from build123d import *

# Parameters (mm, degrees)
EXTRUDE_1_DEPTH     = 5
SKETCH_3_R          = 1.5
CUT_EXTRUDE_1_DEPTH = 5
SKETCH_4_R          = 1.5
CUT_EXTRUDE_2_DEPTH = 50
EXTRUDE_2_DEPTH     = 45
CUT_EXTRUDE_START   = -45
SKETCH_8_R          = 1.5
CUT_EXTRUDE_3_DEPTH = 45


with BuildPart() as part:
    # 草图1 → 凸台-拉伸1 (new body)
    with BuildSketch(Plane(origin=(0, 0, 0), x_dir=(1, 0, 0), z_dir=(0, 1, 0))):
        with BuildLine():
            Line((72.807044649, 44.366167138), (49.314729129, 35.815663555))
            Line((49.314729129, 35.815663555), (49.314729129, 10.486670722))
            Line((49.314729129, 10.486670722), (72.807044649, 1.936167138))
            Line((72.807044649, 1.936167138), (217.807044649, 1.936167138))
            ThreePointArc((217.807044649, 1.936167138), (239.022044649, 23.151167138), (217.807044649, 44.366167138))
            Line((217.807044649, 44.366167138), (72.807044649, 44.366167138))
        make_face()
    extrude(amount=EXTRUDE_1_DEPTH)

    # 草图3 → 切除-拉伸1 (cut)
    with BuildSketch(Plane.XZ):
        with Locations(Location((226.822656109, -14.135555678, 0), (0, 0, 270))):
            Circle(SKETCH_3_R)
        with Locations(Location((224.701335766, -30.045458255, 0), (0, 0, 270))):
            Circle(SKETCH_3_R)
        with Locations(Location((208.791433189, -32.166778599, 0), (0, 0, 270))):
            Circle(SKETCH_3_R)
        with Locations(Location((210.912753532, -16.256876022, 0), (0, 0, 270))):
            Circle(SKETCH_3_R)
    extrude(amount=-CUT_EXTRUDE_1_DEPTH, mode=Mode.SUBTRACT)

    # 草图4 → 切除-拉伸2 (cut)
    with BuildSketch(Plane.XZ):
        with Locations(Location((62.807044649, -11.936167138, 0), (0, 0, 270))):
            Circle(SKETCH_4_R)
        with Locations(Location((52.807044649, -23.151167138, 0), (0, 0, 270))):
            Circle(SKETCH_4_R)
        with Locations(Location((62.807044649, -34.366167138, 0), (0, 0, 270))):
            Circle(SKETCH_4_R)
    extrude(amount=-CUT_EXTRUDE_2_DEPTH, mode=Mode.SUBTRACT)

    # 草图5 → 凸台-拉伸2 (add)
    with BuildSketch(Plane(origin=(0, 5, 0), x_dir=(1, 0, 0), z_dir=(0, 1, 0))):
        Polygon((72.807044649, 44.366167138), (72.807044649, 1.936167138), (49.314729129, 10.486670722), (49.314729129, 35.815663555), align=None)
    extrude(amount=EXTRUDE_2_DEPTH)

    # 草图6 → 切除-放样1 section 0
    with BuildSketch(Plane(origin=(72.807044649, 0, 0), x_dir=(0, 0, -1), z_dir=(1, 0, 0))):
        with BuildLine():
            Line((4.936167138, 5), (4.936167138, 48))
            Line((4.936167138, 48), (41.366167138, 48))
            Line((41.366167138, 48), (41.366167138, 5))
            Line((41.366167138, 5), (4.936167138, 5))
        make_face()
    # 草图7 → 切除-放样1 section 1
    with BuildSketch(Plane.ZY.offset(-49.314729129)):
        with BuildLine():
            Line((-32.839513374, 48), (-32.839513374, 5))
            Line((-32.839513374, 5), (-13.486670722, 5))
            Line((-13.486670722, 5), (-13.486670722, 48))
            Line((-13.486670722, 48), (-32.839513374, 48))
        make_face()
    loft(mode=Mode.SUBTRACT)

    # 草图8 → 切除-拉伸3 (cut)
    with BuildSketch(Plane(origin=(0, 50, 0), x_dir=(1, 0, 0), z_dir=(0, 1, 0)).offset(CUT_EXTRUDE_START)):
        with Locations(Location((62.807044649, 34.366167138, 0), (0, 0, 90))):
            Circle(SKETCH_8_R)
        with Locations(Location((52.807044649, 23.151167138, 0), (0, 0, 90))):
            Circle(SKETCH_8_R)
        with Locations(Location((62.807044649, 11.936167138, 0), (0, 0, 90))):
            Circle(SKETCH_8_R)
    extrude(amount=CUT_EXTRUDE_3_DEPTH, mode=Mode.SUBTRACT)


solid = part.part
The listing builds one solid part. Answer for the finished solid, in the listing's coordinates (mm). A direction names the side the tool comes from. Give positions to 0.01 mm unless a question says otherwise; leave off trailing zeros. Loops run counter-clockwise (first coordinate to the right, second up) from the corner with the lowest first, then second, coordinate; pieces in that order, holes last. Notation, with made-up numbers: (5.25, 44.25) - (46.25, 44.25) arc R24 ccw to (46.25, 59.25) - close; hole circle Ø9 at (14.5, 75.25). An arc over 180 degrees is marked (long way). Write each question's results on one line, items separated by ' | '.
1. Find section A-A, the plane y = 26. Write down the section's boundary in (x, z).
Resolved:
outline: (49.31, -35.82) - (72.81, -44.37) - (72.81, -41.37) - (49.31, -32.84) - close; (49.31, -13.49) - (72.81, -4.94) - (72.81, -1.94) - (49.31, -10.49) - close
2. For a pull along Y with two mould halves and no side action, classify faces 1 (the face through (239.017, 2.465, -22.685)), 2 (the face through (60.9, 26.2, -9.27)), 3 (the face through (143, 0, -23)) as +Y half, -Y half, draft (parallel to the pull), parting line (faces both ways), or undercut.
Resolved:
face 1: draft | face 2: undercut | face 3: -Y half
3. Consider probe 1 along Y at (x, z) = (81.5, -10.5); probe 2 along Y at (x, z) = (59, -20.5); probe 3 along Z at (x, y) = (60.5, 37). Determine where each line is inside the solid, lowest interval first. Write a range as from..to.
Resolved:
probe 1: y = 0..5 | probe 2: y = 0..5, 48..50 | probe 3: z = -39.89..-36.9, -9.42..-6.42
4. Flat-ended cylindrical pins translate along their axes: P1, Ø4, axis at y = 28, z = -36.5, coming from the -X side; P2, Ø3.5, axis at x = 226.82, z = -14.14, coming from the +Y side; P3, Ø21, axis at y = 24, z = -13.5, coming from the +X side. Find the tip coordinate at first contact, or state that the pin passes through.
Resolved:
P1: stops at x = 49.31 | P2: stops at y = 5 | P3: stops at x = 72.81
5. Find section B-B, the plane x = 136.5. Write down the section's boundary in (y, z), then the cut area to 3 significant figures.
Resolved:
outline: (0, -44.37) - (5, -44.37) - (5, -1.94) - (0, -1.94) - close | area: 212 mm^2
6. Which of the six approach directions +Z, -Z, +X, -X, +Y, -Y give full straight-line access (tool end or side, diameter ignored) to faces 4 (the face through (60.896, 26.801, -37.043)), 5 (the face through (144, 2, -1.936)), 6 (the face through (72.807, 49, -23))?
Resolved:
face 4: +X | face 5: +Z, +X, -X, +Y, -Y | face 6: +Z, -Z, +X, +Y
